from build123d import *

# Parameters (mm, degrees)
BOX006_W     = 73.5
BOX006_H     = 11
BOX006_DEPTH = 10
BOX005_W     = 73.5
BOX005_H     = 11
BOX005_DEPTH = 10
BOX004_W     = 88
BOX004_H     = 1
BOX004_DEPTH = 17
BOX003_W     = 88
BOX003_H     = 1
BOX003_DEPTH = 17
BOX002_W     = 88
BOX002_H     = 16.5
BOX002_DEPTH = 39
BOX001_W     = 88
BOX001_H     = 16.5
BOX001_DEPTH = 39
BOX_W        = 90
BOX_H        = 41
BOX_DEPTH    = 43


with BuildPart() as cube006:
    # Box006 → Box006 (new body)
    with BuildSketch(Plane(origin=(8.5, 25.75, 35), x_dir=(1, 0, 0), z_dir=(0, 0, 1))):
        with Locations((36.75, 5.5)):
            Rectangle(BOX006_W, BOX006_H)
    extrude(amount=BOX006_DEPTH)


with BuildPart() as cube005:
    # Box005 → Box005 (new body)
    with BuildSketch(Plane(origin=(8.5, 6.25, 35), x_dir=(1, 0, 0), z_dir=(0, 0, 1))):
        with Locations((36.75, 5.5)):
            Rectangle(BOX005_W, BOX005_H)
    extrude(amount=BOX005_DEPTH)


with BuildPart() as cube004:
    # Box004 → Box004 (new body)
    with BuildSketch(Plane(origin=(0, 38, 2), x_dir=(1, 0, 0), z_dir=(0, 0, 1))):
        with Locations((44, 0.5)):
            Rectangle(BOX004_W, BOX004_H)
    extrude(amount=BOX004_DEPTH)


with BuildPart() as cube003:
    # Box003 → Box003 (new body)
    with BuildSketch(Plane(origin=(0, 18.5, 2), x_dir=(1, 0, 0), z_dir=(0, 0, 1))):
        with Locations((44, 0.5)):
            Rectangle(BOX003_W, BOX003_H)
    extrude(amount=BOX003_DEPTH)


with BuildPart() as cube002:
    # Box002 → Box002 (new body)
    with BuildSketch(Plane(origin=(0, 21.5, 2), x_dir=(1, 0, 0), z_dir=(0, 0, 1))):
        with Locations((44, 8.25)):
            Rectangle(BOX002_W, BOX002_H)
    extrude(amount=BOX002_DEPTH)


with BuildPart() as cube001:
    # Box001 → Box001 (new body)
    with BuildSketch(Plane(origin=(0, 2, 2), x_dir=(1, 0, 0), z_dir=(0, 0, 1))):
        with Locations((44, 8.25)):
            Rectangle(BOX001_W, BOX001_H)
    extrude(amount=BOX001_DEPTH)


with BuildPart() as cut005:
    # Box → Box (new body)
    with BuildSketch(Plane.XY):
        with Locations((45, 20.5)):
            Rectangle(BOX_W, BOX_H)
    extrude(amount=BOX_DEPTH)

    # Cut: cut Cube001
    add(cube001.part, mode=Mode.SUBTRACT)

    # Cut001: cut Cube002
    add(cube002.part, mode=Mode.SUBTRACT)

    # Cut002: cut Cube003
    add(cube003.part, mode=Mode.SUBTRACT)

    # Cut003: cut Cube004
    add(cube004.part, mode=Mode.SUBTRACT)

    # Cut004: cut Cube005
    add(cube005.part, mode=Mode.SUBTRACT)

    # Cut005: cut Cube006
    add(cube006.part, mode=Mode.SUBTRACT)


solid = cut005.part
CAD build for the part. Positions are in the model's coordinates, mm. A direction names the side the tool comes from. Coordinates: 2 decimals unless noted, no trailing zeros. Write each loop counter-clockwise with the first axis right and the second up, starting at its lowest first coordinate (ties: lowest second). Pieces come first, ordered by that corner, then holes. Notation, with made-up numbers: M 31,22 L 62,22 A24 cw 62,32 Z; hole C 80,77 d3. An arc over 180 degrees is marked long. Return JSON: item names as keys, results as strings.
Item 1: Which spindle directions (+Z, -Z, +X, -X, +Y, -Y) get a long thin tool onto all of the face, cutting with end or side? Do faces 1 (the flat face through (90, 20, 21)), 2 (the flat face through (45, 6.25, 42)), 3 (the flat face through (43, 19.5, 10)). Say none if no direction does.
Findings below:
{"face 1": "+Z, -Z, +X, +Y, -Y", "face 2": "+Z", "face 3": "-X"}
Item 2: Slice it at B-B, the plane x = 6. Write the cut outline in (y, z).
Findings below:
{"outline": "M 0,0 L 41,0 L 41,43 L 0,43 Z; hole M 2,2 L 19.5,2 L 19.5,19 L 18.5,19 L 18.5,41 L 2,41 Z; hole M 21.5,2 L 39,2 L 39,19 L 38,19 L 38,41 L 21.5,41 Z"}
Item 3: Slice it at A-A, the plane y = 34.5. Write the cut outline in (x, z).
Findings below:
{"outline": "M 0,0 L 90,0 L 90,43 L 82,43 L 82,41 L 88,41 L 88,2 L 0,2 Z; M 0,41 L 8.5,41 L 8.5,43 L 0,43 Z"}
Item 4: Slice it at D-D, the plane y = 24.5. Write the cut outline in (x, z).
Findings below:
{"outline": "M 0,0 L 90,0 L 90,43 L 0,43 L 0,41 L 88,41 L 88,2 L 0,2 Z"}
Item 5: Two-plate mould, pull along Z, no slides. Class faces 4 (the flat face through (43, 5, 41)), 5 (the flat face through (45, 36.75, 42)), 6 (the flat face through (44, 21, 43)), 7 (the flat face through (44, 21, 0)): +Z half, -Z half, draft (parallel to the pull), parting line (faces both ways), or undercut.
Findings below:
{"face 4": "undercut", "face 5": "draft", "face 6": "+Z half", "face 7": "-Z half"}
Item 6: Slice it at C-C, the plane z = 29.5. Write the cut outline in (x, y), and give its area (3 significant figures).
Findings below:
{"outline": "M 0,0 L 90,0 L 90,41 L 0,41 L 0,38 L 88,38 L 88,21.5 L 0,21.5 L 0,18.5 L 88,18.5 L 88,2 L 0,2 Z", "area": "786 mm2"}
Item 7: Drop flat-ended pins along their axis: pin 1 Ø3 at (x, y) = (16.5, 33.5) entering from +Z; pin 2 Ø5 at (y, z) = (26.5, 28) entering from -X. Give the stop position or say it passes through.
Findings below:
{"pin 1": "stops at z = 2", "pin 2": "stops at x = 88"}
Item 8: Probe line 1 (Y direction, x = 4, z = 7.5); line 2 (Y direction, x = 78.5, z = 29); line 3 (Z direction, x = 76.5, y = 37). List the from-to ranges inside material, lowest first. Write a range as from..to.
Findings below:
{"line 1": "y = 0..2, 19.5..21.5, 39..41", "line 2": "y = 0..2, 18.5..21.5, 38..41", "line 3": "z = 0..2, 41..43"}
